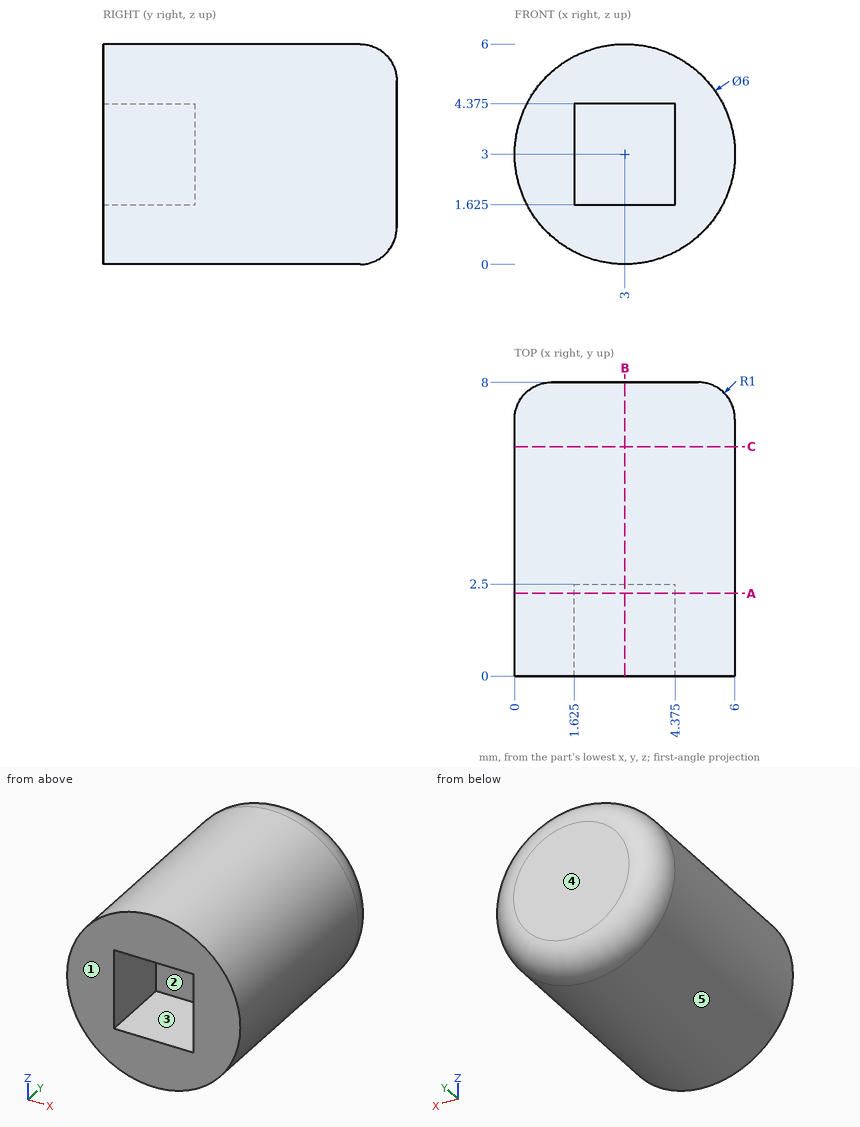
For this review, use the dimensioned drawing (mm, ordinates from the lowest corner) and the shaded views. A direction names the side the tool comes from. Coordinates: 2 decimals unless noted, no trailing zeros. Loops run counter-clockwise (first coordinate to the right, second up) from the corner with the lowest first, then second, coordinate; pieces in that order, holes last. Notation, with made-up numbers: (-26.5, 60) -> (-22.5, 60) arc R9 ccw to (-22.5, 69) -> close; hole circle Ø3 at (14, -36.5). An arc over 180 degrees is marked (long way). Use a Markdown table: item, result. Add a question column.
Item 1: Clearance check with flat-ended pins moving along their axes: P1, Ø3, axis at y = 1.5, z = 2.5, coming from the -X side; P2, Ø1.4, axis at x = 3, z = 2.5, coming from the -Y side. State where each tip first meets the part, or that it passes through.
Item 2: Machinability: for the marked faces 1 and 2, which of the approach directions +Z, -Z, +X, -X, +Y, -Y give a long, thin tool a straight path to every point of the face, cutting with its end or side? Answer none if there is none.
Item 3: We need section C-C, the plane y = 6.25. Write out the cut boundary in (x, z).
Item 4: Wall thickness on L1, parallel to X at y = 2, z = 2 (3 decimals); L2, parallel to X at y = 1, z = 1.75 (3 decimals); L3, parallel to Z at x = 4.3, y = 0.75 (3 decimals): over which ranges is each line inside the solid? List them lowest first. Write a range as from..to.
Item 5: We need section A-A, the plane y = 2.25. Write out the cut boundary in (x, z) (3 decimals).
Item 6: We need section B-B, the plane x = 3. Write out the cut boundary in (y, z) (3 decimals).
Item 7: The part is to be moulded in two halves that separate along X. For the marked faces 3, 4 and 5, say which applies: +X half, -X half, draft (parallel to the pull), parting line (faces both ways), or undercut.
Numbers:
| question | item | result |
|---|---|---|
| 1 | P1 | stops at x = 0 |
| 1 | P2 | stops at y = 2.5 |
| 2 | face 1 | +Z, -Z, +X, -X, -Y |
| 2 | face 2 | -Y |
| 3 | outline | circle Ø6 at (3, 3) |
| 4 | L1 | x = 0.172..1.625, 4.375..5.828 |
| 4 | L2 | x = 0.273..1.625, 4.375..5.727 |
| 4 | L3 | z = 0.296..1.625, 4.375..5.704 |
| 5 | outline | circle Ø6 at (3, 3); hole (1.625, 1.625) -> (4.375, 1.625) -> (4.375, 4.375) -> (1.625, 4.375) -> close |
| 6 | outline | (0, 0) -> (7, 0) arc R1 ccw to (8, 1) -> (8, 5) arc R1 ccw to (7, 6) -> (0, 6) -> (0, 4.375) -> (2.5, 4.375) -> (2.5, 1.625) -> (0, 1.625) -> close |
| 7 | face 3 | undercut |
| 7 | face 4 | draft |
| 7 | face 5 | parting line |
